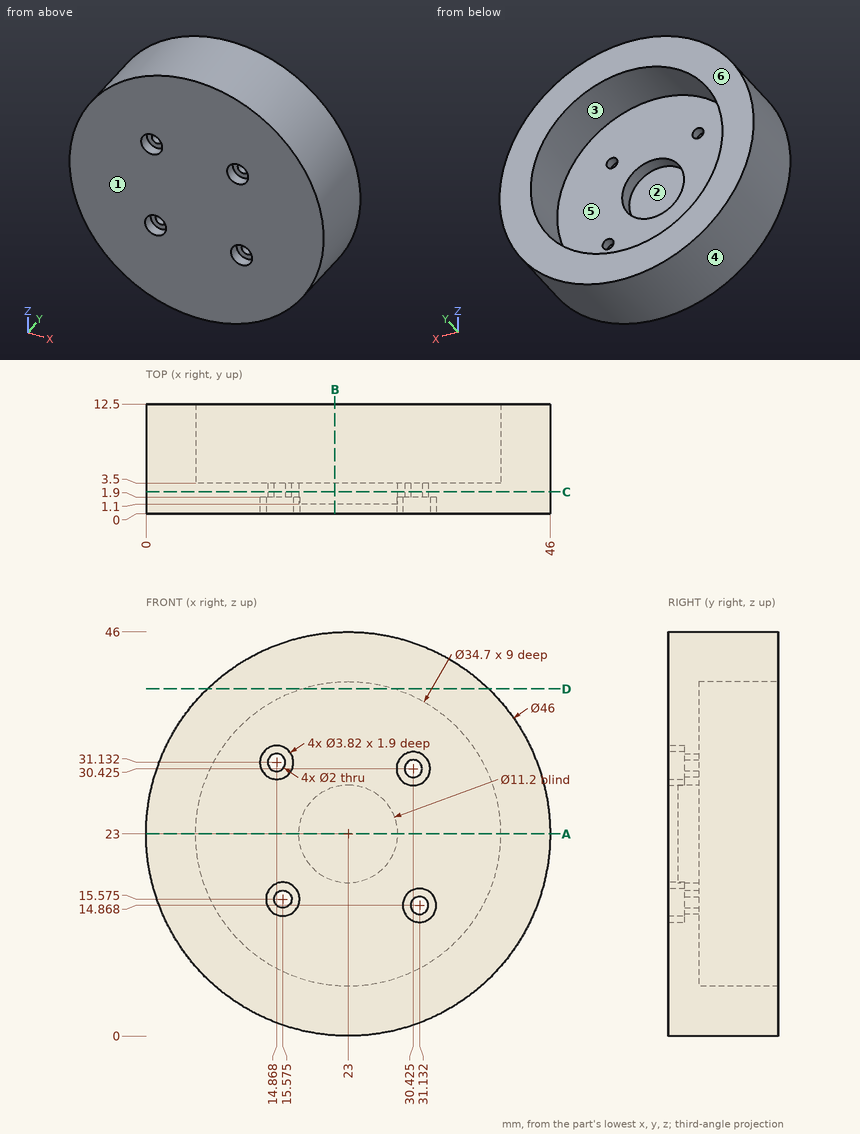
Print and shaded views of the part. All mm, measured from the part's lowest x, y and z. A direction names the side the tool comes from. Coordinates: 2 decimals unless noted, no trailing zeros. Write each loop counter-clockwise with the first axis right and the second up, starting at its lowest first coordinate (ties: lowest second). Pieces come first, ordered by that corner, then holes.
(1) Cut at D-D, the plane z = 39.5. List the corners of the cut face in (x, y), and give its area (3 significant figures).
(2) Two-plate mould, pull along Z, no slides. Class the marked faces 3, 4, 5 and 6: +Z half, -Z half, draft (parallel to the pull), parting line (faces both ways), or undercut.
(3) Cut at B-B, the plane x = 21.5. List the corners of the cut face in (y, z) (1 decimal).
(4) Cut at C-C, the plane y = 2.5. List the corners of the cut face in (x, z) (1 decimal), and give its area (3 significant figures).
(5) 3-axis set-ups, long thin cutter, end or side, ignore diameter. For the marked faces 1 and 2: which of +Z, -Z, +X, -X, +Y, -Y reach the whole face in a straight line?
(6) Cut at A-A, the plane z = 23. List the corners of the cut face in (x, y).
(7) Drill centre lines: probe 1 along X at (y, z) = (1.75, 23); probe 2 along Y at (x, z) = (21, 16.5); probe 3 along Z at (x, y) = (27.5, 6.25) (1 decimal). Where is each one in solid material? Low to high.
(8) Flat gauge pins, fed straight in: pin 1 (10.5 mm diameter, centred on x = 17, z = 29, fed in from +Y); pin 2 (4 mm diameter, centred on x = 31, z = 29.5, fed in from -Y); pin 3 (1.9 mm diameter, centred on x = 15.5, z = 30.5, fed in from -Y); pin 4 (4 mm diameter, centred on y = 2.5, z = 41, fed in from -X). Where does each tip first touch, or does it go through?
Geometry says:
1. outline: (6.98, 0) - (39.02, 0) - (39.02, 12.5) - (28.36, 12.5) - (28.36, 3.5) - (17.64, 3.5) - (17.64, 12.5) - (6.98, 12.5) - close
1. area: 304 mm2
2. face 3: undercut
2. face 4: parting line
2. face 5: undercut
2. face 6: draft
3. outline: (0, 0) - (12.5, 0) - (12.5, 5.7) - (3.5, 5.7) - (3.5, 17.6) - (1.1, 17.6) - (1.1, 28.4) - (3.5, 28.4) - (3.5, 40.3) - (12.5, 40.3) - (12.5, 46) - (0, 46) - close
4. outline: circle Ø46 at (23, 23); hole circle Ø2 at (14.9, 31.1); hole circle Ø2 at (15.6, 15.6); hole circle Ø11.2 at (23, 23); hole circle Ø2 at (30.4, 30.4); hole circle Ø2 at (31.1, 14.9)
4. area: 1,550 mm2
5. face 1: +Z, -Z, +X, -X, -Y
5. face 2: +Y
6. outline: (0, 0) - (46, 0) - (46, 12.5) - (40.35, 12.5) - (40.35, 3.5) - (28.6, 3.5) - (28.6, 1.1) - (17.4, 1.1) - (17.4, 3.5) - (5.65, 3.5) - (5.65, 12.5) - (0, 12.5) - close
7. probe 1: x = 0 to 17.4, 28.6 to 46
7. probe 2: y = 0 to 3.5
7. probe 3: z = 0.4 to 6.2, 39.8 to 45.6
8. pin 1: stops at y = 3.5
8. pin 2: stops at y = 0
8. pin 3: stops at y = 1.9
8. pin 4: stops at x = 6.48
